Can you work these out from the model? Positions are in its coordinate system, mm. Face numbers are marked on the shaded views. Coordinates: 2 decimals unless noted, no trailing zeros. Loops run counter-clockwise (first coordinate to the right, second up) from the corner with the lowest first, then second, coordinate; pieces in that order, holes last.
Autodesk Inventor part; units mm, degrees
ref_plane "YZ Plane" through (0, 0, 0) normal (1, 0, 0) x (0, 1, 0)
ref_plane "XZ Plane" through (0, 0, 0) normal (0, 1, 0) x (-1, 0, 0)
ref_plane "XY Plane" through (0, 0, 0) normal (0, 0, 1) x (1, 0, 0)
sketch "Sketch1" plane through (0, 0, 0) normal (0, 1, 0) x (-1, 0, 0)
  line L0 (43.4289, -18.5999) -> (-45.4711, -18.5999)
  line L1 (-45.4711, -18.5999) -> (-45.4711, 24.5801)
  line L2 (-45.4711, 24.5801) -> (43.4289, 24.5801)
  line L3 (43.4289, 24.5801) -> (43.4289, -18.5999)
  point P0 (0, 0)
  dimension "d2" = 88.9
  dimension "d3" = 43.18
extrude "Extrusion1" add sketch "Sketch1" along normal blind 6.35
sketch "Sketch2" plane through (0, 6.35, 0) normal (0, 1, 0) x (1, 0, 0)
  line L0 (45.4711, -24.5801) -> (45.4711, 18.5999)
  line L1 (45.4711, 18.5999) -> (-43.4289, 18.5999)
  point P0 (0, 0)
  point P1 (1.0211, -24.5835)
  dimension "d22" = 44.45
  dimension "d23" = 43.1834
hole "Hole1" at (1.0211, 6.35, 24.5835) direction (0, -1, 0) diameter 41.148 end through all
sketch "Sketch3" plane through (0, 6.35, 0) normal (0, 1, 0) x (1, 0, 0)
  line L0 (-43.4289, 18.5999) -> (-43.4289, -24.5801)
  line L1 (-43.4289, -24.5801) -> (-19.5529, -24.5801)
  point P0 (0, 0)
  point P1 (-30.7289, -11.8801)
  dimension "d13" = 12.7
  dimension "d14" = 12.7
hole "Hole2" at (-30.7289, 6.35, 11.8801) direction (0, -1, 0) diameter 4.826 end through all
sketch "Sketch4" plane through (0, 6.35, 0) normal (0, 1, 0) x (1, 0, 0)
  line L0 (45.4711, 18.5999) -> (-43.4289, 18.5999)
  line L1 (45.4711, -24.5801) -> (45.4711, 18.5999)
  point P0 (0, 0)
  point P1 (1.0211, 5.8999)
  dimension "d24" = 12.7
  dimension "d25" = 44.45
hole "Hole3" at (1.0211, 6.35, -5.8999) direction (0, -1, 0) diameter 4.826 end through all
properties part number "InventorPart1Commit3"
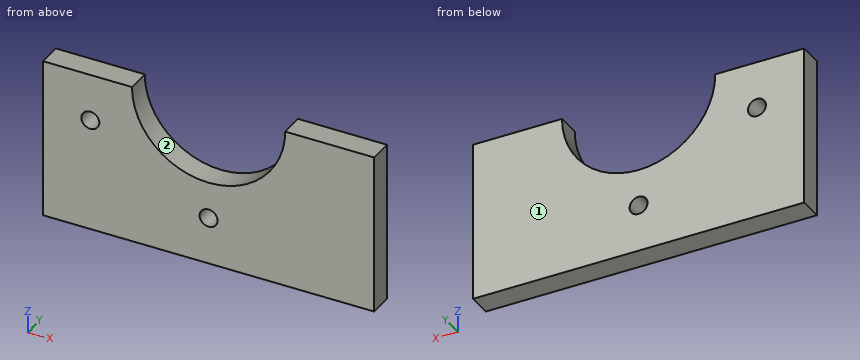
Item 1: Suppose I cut it at A-A, the plane z = -6.5. Please give me the cut outline in (x, y), plus the area to 3 significant figures.
Results are:
outline: (-43.43, 0) - (-1.32, 0) - (-1.32, 6.35) - (-43.43, 6.35) - close; (3.36, 0) - (45.47, 0) - (45.47, 6.35) - (3.36, 6.35) - close
area: 535 mm2
Item 2: Suppose I cut it at B-B, the plane x = 2. Please give me the cut outline in (y, z).
Results are:
outline: (0, -18.6) - (6.35, -18.6) - (6.35, -8.11) - (0, -8.11) - close; (0, -3.69) - (6.35, -3.69) - (6.35, 4.03) - (0, 4.03) - close
Item 3: Suppose I cut it at D-D, the plane x = -13. Please give me the cut outline in (y, z), plus the area to 3 significant figures.
Results are:
outline: (0, -18.6) - (6.35, -18.6) - (6.35, 9.53) - (0, 9.53) - close
area: 179 mm2
Item 4: We'd pull the mould along X, two halves only. Please class the marked faces 1 and 2: +X half, -X half, draft (parallel to the pull), parting line (faces both ways), or undercut.
Results are:
face 1: draft
face 2: undercut
Item 5: I need wall thicknesses on line 1 along X through (y, z) = (5.5, 13); line 2 along X through (y, z) = (3.5, 15); line 3 along X through (y, z) = (2.5, -4.5). Which ranges of each line are inside material? Lowest first, please.
Results are:
line 1: x = -43.43 to -32.87, -28.59 to -15.98, 18.02 to 45.47
line 2: x = -43.43 to -17.18, 19.23 to 45.47
line 3: x = -43.43 to -0.94, 2.99 to 45.47
Item 6: Suppose I cut it at C-C, the plane y = 5. Please give me the cut outline in (x, z), plus the area to 3 significant figures.
Results are:
outline: (-43.43, -18.6) - (45.47, -18.6) - (45.47, 24.58) - (21.6, 24.58) arc R20.57 cw to (-19.55, 24.58) - (-43.43, 24.58) - close; hole circle Ø4.83 at (-30.73, 11.88); hole circle Ø4.83 at (1.02, -5.9)
area: 3,140 mm2
